For this review, take the finished solid that the model builds, in its own axes (mm). Give positions to 0.01 mm unless a question says otherwise; leave off trailing zeros. Order: outer loops, then holes, each group sorted by start corner. A loop starts at its lowest first (then second) coordinate and runs counter-clockwise, first axis right, second up. Notation, with made-up numbers: M -3,20.5 L 35,20.5 A22 ccw 35,58.5 Z; hole C 5.5,34 d11. An arc over 180 degrees is marked long. Use CSV: the item, a comma, the result in double quotes. Start each with the question number.
(1) Wall thickness on L1, parallel to Z at x = 4, y = 4.75; L2, parallel to Y at x = -73, z = -94.5; L3, parallel to Z at x = 47, y = 1: over which ranges is each line inside the solid? List them lowest first. Write a range as from..to.
(2) Clearance check with flat-ended pins moving along their axes: P1, Ø1.2, axis at y = 5.5, z = 0, coming from the +X side; P2, Ø1.6, axis at x = -5.5, y = 5, coming from the -Z side; P3, Ø8, axis at x = -87, z = -98, coming from the +Y side; P4, Ø1, axis at x = 77.5, y = 3.5, coming from the +Z side. State where each tip first meets the part, or that it passes through.
(3) Consider section C-C (x = -127). Write out the cut boundary in (y, z).
(4) Consider section A-A (x = 0). Write out the cut boundary in (y, z).
(5) Consider section B-B (z = -101). Write out the cut boundary in (x, y).
```python
from build123d import *

# Parameters (mm, degrees)
ESQUISSE1_R             = 150
BOSS_EXTRU_1_DEPTH      = 2
ESQUISSE2_W             = 2
ESQUISSE2_H             = 13.5
ESQUISSE2_W_2           = 9.5
BOSS_EXTRU_2_DEPTH      = 7
ENL_V_MAT_EXTRU_2_DEPTH = 30
ENL_V_MAT_EXTRU_3_DEPTH = 9.5
ENL_V_MAT_EXTRU_4_DEPTH = 213.172624294


with BuildPart() as part:
    # Esquisse1 → Boss.-Extru.1 (new body)
    with BuildSketch(Plane(origin=(0, 0, 0), x_dir=(1, 0, 0), z_dir=(0, 1, 0))):
        with Locations(Location((0, 0, 0), (0, 0, 270))):
            Circle(ESQUISSE1_R)
    extrude(amount=BOSS_EXTRU_1_DEPTH)

    # Esquisse2 → Boss.-Extru.2 (add)
    with BuildSketch(Plane(origin=(0, 2, 0), x_dir=(1, 0, 0), z_dir=(0, 1, 0))):
        with Locations((-5.75, 0)):
            Rectangle(ESQUISSE2_W, ESQUISSE2_H)
        Rectangle(ESQUISSE2_W_2, ESQUISSE2_H)
    extrude(amount=BOSS_EXTRU_2_DEPTH)

    # Esquisse3 → Enl_v. mat.-Extru.2 (cut)
    with BuildSketch(Plane(origin=(4.75, 0, 0), x_dir=(0, 0, -1), z_dir=(1, 0, 0))):
        Polygon((-6, 2), (-6, 6.15), (-1.65, 6.15), (1.65, 6.15), (6, 6.15), (6, 2), (6.75, 2), (6.75, 9), (-6.75, 9), (-6.75, 2), align=None)
    extrude(amount=-ENL_V_MAT_EXTRU_2_DEPTH, mode=Mode.SUBTRACT)

    # Esquisse3_3 → Enl_v. mat.-Extru.3 (cut)
    with BuildSketch(Plane(origin=(4.75, 0, 0), x_dir=(0, 0, -1), z_dir=(1, 0, 0))):
        with BuildLine():
            ThreePointArc((-1.246071429, 5.0684243), (-4.054607326, 3.712293965), (-6, 6.15))
            Line((-6, 6.15), (-6, 2))
            Line((-6, 2), (6, 2))
            Line((6, 2), (6, 6.15))
            ThreePointArc((6, 6.15), (4.054607326, 3.712293965), (1.246071429, 5.0684243))
            ThreePointArc((1.246071429, 5.0684243), (0, 4.5), (-1.246071429, 5.0684243))
        make_face()
    extrude(amount=-ENL_V_MAT_EXTRU_3_DEPTH, mode=Mode.SUBTRACT)

    # Esquisse4 → Enl_v. mat.-Extru.4 (cut, through all)
    with BuildSketch(Plane(origin=(0, 2, 0), x_dir=(1, 0, 0), z_dir=(0, 1, 0))):
        with BuildLine():
            Line((-90, -120), (90, -120))
            ThreePointArc((90, -120), (0, -150), (-90, -120))
        make_face()
    extrude(amount=-ENL_V_MAT_EXTRU_4_DEPTH, mode=Mode.SUBTRACT)


solid = part.part
```
Check result:
1,L1,"z = -5.57..-1.43, -0.87..0.87, 1.43..5.57"
1,L2,"y = 0..2"
1,L3,"z = -142.45..120"
2,P1,"stops at x = 4.75"
2,P2,"stops at z = -6"
2,P3,"stops at y = 2"
2,P4,"passes through"
3,outline,"M 0,-79.82 L 2,-79.82 L 2,79.82 L 0,79.82 Z"
4,outline,"M 0,-150 L 2,-150 L 2,120 L 0,120 Z; M 5.07,-1.25 A2.5 ccw 6.15,-6 L 6.15,6 A2.5 ccw 5.07,1.25 A1.65 ccw Z"
5,outline,"M -110.9,0 L 110.9,0 L 110.9,2 L -110.9,2 Z"
